Part model, mm, in its own coordinate system. A direction names the side the tool comes from. Coordinates: 2 decimals unless noted, no trailing zeros. Loops run counter-clockwise (first coordinate to the right, second up) from the corner with the lowest first, then second, coordinate; pieces in that order, holes last. Notation, with made-up numbers: M -2.75,-21.5 L 47.25,-21.5 A24 ccw 47.25,8.5 Z; hole C 19,-6 d4. An arc over 180 degrees is marked long. Answer as CSV lines item,"result". Start each with the question number.
from build123d import *

# Parameters (mm, degrees)
SKETCH_R        = 3.5
SKETCH_R_2      = 1.6
PAD_DEPTH       = 1.2
SKETCH001_W     = 119.586
SKETCH001_H     = 17.78
SKETCH001_R     = 1.6
PAD001_DEPTH    = 1.5
SKETCH002_R     = 3.5
SKETCH002_R_2   = 1.6
PAD002_DEPTH    = 1.2
SKETCH003_R     = 1.6
POCKET_DEPTH    = 2.701
PAD003_DEPTH    = 17.78
CHAMFER_SIZE    = 2.2
CHAMFER002_SIZE = 0.6


with BuildPart() as part:
    # Sketch (on Face1 of CopyPcb_f5c5) → Pad (new body)
    with BuildSketch(Plane(origin=(-93.484762, 101.426, -1.6), x_dir=(1, 0, 0), z_dir=(0, 0, -1))):
        with Locations((113.233762, 92.79)):
            Circle(SKETCH_R)
        with Locations((113.233762, 92.79)):
            Circle(SKETCH_R_2, mode=Mode.SUBTRACT)
    extrude(amount=PAD_DEPTH)

    # Sketch001 (on Face4 of Pad) → Pad001 (join)
    with BuildSketch(Plane(origin=(-93.484762, 101.426, -2.8), x_dir=(1, 0, 0), z_dir=(0, 0, -1))):
        with Locations((153.277762, 92.79)):
            Rectangle(SKETCH001_W, SKETCH001_H)
        with Locations((113.233762, 92.79)):
            Circle(SKETCH001_R, mode=Mode.SUBTRACT)
    extrude(amount=PAD001_DEPTH)

    # Sketch002 (on Face3 of Pad001) → Pad002 (join)
    with BuildSketch(Plane(origin=(-93.484762, 101.426, -2.8), x_dir=(1, 0, 0), z_dir=(0, 0, 1))):
        with Locations((160.733762, -92.79)):
            Circle(SKETCH002_R)
        with Locations((160.733762, -92.79)):
            Circle(SKETCH002_R_2, mode=Mode.SUBTRACT)
    extrude(amount=PAD002_DEPTH)

    # Sketch003 (on Face11 of Pad002) → Pocket (cut, through all)
    with BuildSketch(Plane(origin=(-93.484762, 101.426, -4.3), x_dir=(1, 0, 0), z_dir=(0, 0, -1))):
        with Locations((160.733762, 92.79)):
            Circle(SKETCH003_R)
    extrude(amount=-POCKET_DEPTH, mode=Mode.SUBTRACT)

    # Sketch004 (on Face6 of Pocket) → Pad003 (join)
    with BuildSketch(Plane(origin=(-93.484762, -0.254, -1.6), x_dir=(1, 0, 0), z_dir=(0, -1, 0))):
        with BuildLine():
            Line((202.656762, -1.2), (205.456762, 1.6))
            Line((205.456762, 1.6), (213.070762, 1.6))
            Line((213.070762, 1.2), (213.070762, 1.6))
            ThreePointArc((213.070762, 1.2), (212.070762, 0.2), (213.070762, -0.8))
            Line((213.070762, -0.8), (213.070762, -1.2))
            Line((213.070762, -1.2), (202.656762, -1.2))
        make_face()
    extrude(amount=-PAD003_DEPTH)

    # Chamfer
    chamfer_edges = [part.edges().sort_by_distance(p)[0] for p in [
        (18.149, 8.636, -4.3),
        (65.649, 8.636, -4.3),
    ]]
    chamfer(chamfer_edges, length=CHAMFER_SIZE)

    # Chamfer002
    chamfer002_edges = [part.edges().sort_by_distance(p)[0] for p in [
        (16.249, 8.636, -2.8),
        (63.749, 8.636, -2.8),
    ]]
    chamfer(chamfer002_edges, length=CHAMFER002_SIZE)


solid = part.part
Q1. Flat gauge pins, fed straight in: P1, Ø4, axis at x = 57.5, y = 12, coming from the +Z side; P2, Ø5.5, axis at x = 67, y = 8, coming from the +Z side; P3, Ø2, axis at y = 14, z = -0.5, coming from the -X side. Where does each tip first touch, or does it go through?
Q2. Tool access for faces 4 (the face through (110.55, 8.51, -1.42)), 5 (the face through (23.087, 7.585, -1.896)), 6 (the face through (68, 7, -1.6)), 7 (the face through (20.487, 10.055, -1.846)): list every direction of +Z, -Z, +X, -X, +Y, -Y with a clear straight run to the whole face (end or side of a thin tool).
Q3. Wall check: L1, parallel to X at y = 8.25, z = -2.3; L2, parallel to Z at x = 34, y = 2.75; L3, parallel to X at y = 8, z = -3.95. Give the ranges that are in metal, low to high.
Q4. Two-plate mould, pull along X, no slides. Class faces 1 (the face through (21.38, 8.12, -2.21)), 2 (the face through (118.586, 8.512, -1.378)), 3 (the face through (18, 9, -1.6)): +X half, -X half, draft (parallel to the pull), parting line (faces both ways), or undercut.
Q5. Slice it at B-B, the plane x = 41. Write the cut outline in (y, z), and give its area (3 significant figures).
Q6. Slice it at A-A, the plane y = 3.25. Write the cut outline in (x, z).
Solved:
1,P1,"stops at z = -2.8"
1,P2,"stops at z = -1.6"
1,P3,"stops at x = 110.47"
2,face 4,"+Z, +Y, -Y"
2,face 5,"+Z"
2,face 6,"+Z, -X, +Y, -Y"
2,face 7,"+Z, -Z"
3,L1,"x = 16.17 to 17.99, 21.51 to 23.33, 63.67 to 65.49, 69.01 to 70.83, 109.67 to 119.15"
3,L2,"z = -4.3 to -2.8"
3,L3,"x = 0 to 16.36, 23.14 to 63.86, 70.64 to 119.59"
4,face 1,"undercut"
4,face 2,"+X half"
4,face 3,"draft"
5,outline,"M -0.25,-4.3 L 17.53,-4.3 L 17.53,-2.8 L -0.25,-2.8 Z"
5,area,"26.7 mm2"
6,outline,"M 0,-4.3 L 119.59,-4.3 L 119.59,-2.4 A1 cw 119.59,-0.4 L 119.59,0 L 111.97,0 L 109.17,-2.8 L 0,-2.8 Z"
